from build123d import *

# Parameters (mm, degrees)
EXTRUDE_1_DEPTH     = 77
SKETCH_2_R          = 1.75
CUT_EXTRUDE_1_DEPTH = 20
SKETCH_3_W          = 6
SKETCH_3_H          = 3
CUT_EXTRUDE_2_DEPTH = 84.228292678
SKETCH_4_R          = 13.25
CUT_EXTRUDE_3_DEPTH = 84.228292678
SKETCH_7_R          = 1.75
CUT_EXTRUDE_4_DEPTH = 84.228292822


with BuildPart() as part:
    # Эскиз1 → Бобышка-Вытянуть1 (new body)
    with BuildSketch(Plane(origin=(0, 0, 0), x_dir=(-1, 0, 0), z_dir=(0, 1, 0))):
        with BuildLine():
            Line((27.5, 9.103890562), (20.77355029, -2.54666209))
            ThreePointArc((20.77355029, -2.54666209), (0, 0), (-20.77355029, -2.54666209))
            Line((-20.77355029, -2.54666209), (-27.5, 9.103890562))
            ThreePointArc((-27.5, 9.103890562), (0, 13), (27.5, 9.103890562))
        make_face()
    extrude(amount=EXTRUDE_1_DEPTH)

    # Эскиз2 → Вырез-Вытянуть1 (cut)
    with BuildSketch(Plane.XZ):
        with Locations(Location((0, 6.5, 0), (0, 0, 270))):
            Circle(SKETCH_2_R)
        with Locations(Location((16.059644847, 5.07877185, 0), (0, 0, 270))):
            Circle(SKETCH_2_R)
        with Locations(Location((-16.059644847, 5.07877185, 0), (0, 0, 270))):
            Circle(SKETCH_2_R)
    extrude(amount=-CUT_EXTRUDE_1_DEPTH, mode=Mode.SUBTRACT)

    # Эскиз3 → Вырез-Вытянуть2 (cut, through all)
    with BuildSketch(Plane.XY.offset(13)):
        with Locations((-16.059644847, 11.5)):
            Rectangle(SKETCH_3_W, SKETCH_3_H)
        with Locations((0, 11.5)):
            Rectangle(SKETCH_3_W, SKETCH_3_H)
        with Locations((16.059644847, 11.5)):
            Rectangle(SKETCH_3_W, SKETCH_3_H)
    extrude(amount=-CUT_EXTRUDE_2_DEPTH, mode=Mode.SUBTRACT)

    # Эскиз4 → Вырез-Вытянуть3 (cut, through all)
    with BuildSketch(Plane.XY.offset(13)):
        with Locations((0, 44.5)):
            Circle(SKETCH_4_R)
    extrude(amount=-CUT_EXTRUDE_3_DEPTH, mode=Mode.SUBTRACT)

    # Эскиз7 → Вырез-Вытянуть4 (cut, through all)
    with BuildSketch(Plane.XY.offset(13)):
        with Locations((-17.5, 62)):
            Circle(SKETCH_7_R)
        with Locations((17.5, 62)):
            Circle(SKETCH_7_R)
        with Locations((17.5, 27)):
            Circle(SKETCH_7_R)
        with Locations((-17.5, 27)):
            Circle(SKETCH_7_R)
    extrude(amount=-CUT_EXTRUDE_4_DEPTH, mode=Mode.SUBTRACT)


solid = part.part
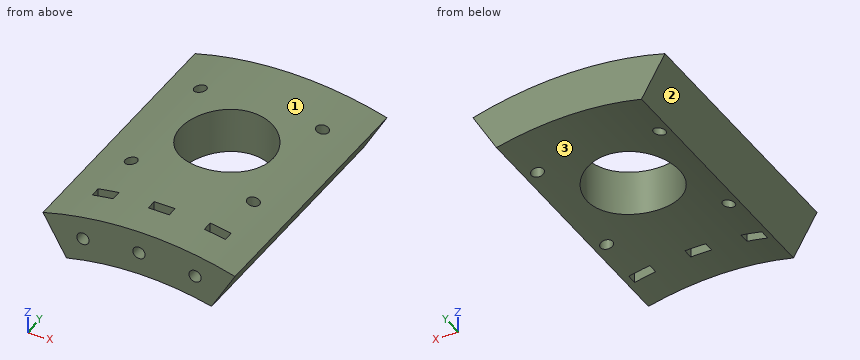
Part model, mm, in its own coordinate system. Face numbers are marked on the shaded views. Coordinates: 2 decimals unless noted, no trailing zeros. Order: outer loops, then holes, each group sorted by start corner. A loop starts at its lowest first (then second) coordinate and runs counter-clockwise, first axis right, second up.
(1) Pull direction X, two halves, no side cores. Call the marked faces 1, 2 and 3: pulls with the +X half, pulls with the -X half, needs draft (parallel to the pull), parting line crosses it, or undercut.
Check sheet entries:
face 1: parting line crosses it
face 2: pulls with the -X half
face 3: undercut
(2) Slice it at D-D, the plane z = 1.5. State how many separate pieces and enclosed holes the cut face has, and give its area (3 significant figures).
Check sheet entries:
separate pieces: 1
enclosed holes: 8
area: 2,910 mm2
(3) Slice it at A-A, the plane x = 0. Write the cut outline in (y, z).
Check sheet entries:
outline: (0, 0) - (10, 0) - (10, 4.75) - (0, 4.75) - close; (0, 8.25) - (10, 8.25) - (10, 13) - (0, 13) - close; (13, 0) - (31.25, 0) - (31.25, 13) - (13, 13) - (13, 8.25) - (20, 8.25) - (20, 4.75) - (13, 4.75) - close; (57.75, 0) - (77, 0) - (77, 13) - (57.75, 13) - close
(4) Probe L1, parallel to Y at x = -13.5, z = 2.75; L2, parallel to X at y = 13.5, z = 5.25; L3, parallel to Y at x = 18, z = 2.25. List the from-to ranges inside material, lowest first.
Check sheet entries:
L1: y = 0 to 10, 13 to 77
L2: x = -25.27 to -17.8, -14.32 to -1.22, 1.22 to 14.32, 17.8 to 25.27
L3: y = 0 to 10, 13 to 25.32, 28.68 to 60.32, 63.68 to 77
(5) Slice it at B-B, the plane y = 62. Write the cut outline in (x, z), and give its area (3 significant figures).
Check sheet entries:
outline: (-27.5, 9.1) - (-20.77, -2.55) arc R86 cw to (-19.25, -2.18) - (-19.25, 11.11) arc R99 ccw to start; (-15.75, -1.45) arc R86 cw to (15.75, -1.45) - (15.75, 11.74) arc R99 ccw to (-15.75, 11.74) - close; (19.25, -2.18) arc R86 cw to (20.77, -2.55) - (27.5, 9.1) arc R99 ccw to (19.25, 11.11) - close
area: 542 mm2
(6) Slice it at C-C, the plane x = -17. Write the cut outline in (y, z), and give its area (3 significant figures).
Check sheet entries:
outline: (0, -1.7) - (10, -1.7) - (10, 3.6) - (0, 3.6) - close; (0, 6.55) - (10, 6.55) - (10, 11.53) - (0, 11.53) - close; (13, -1.7) - (25.32, -1.7) - (25.32, 11.53) - (13, 11.53) - (13, 6.55) - (20, 6.55) - (20, 3.6) - (13, 3.6) - close; (28.68, -1.7) - (60.32, -1.7) - (60.32, 11.53) - (28.68, 11.53) - close; (63.68, -1.7) - (77, -1.7) - (77, 11.53) - (63.68, 11.53) - close
area: 840 mm2
(7) Pin check, flat tips, straight feed: pin 1 Ø1.5 at (y, z) = (11, 5) entering from -X; pin 2 Ø3 at (x, y) = (17.5, 62) entering from +Z; pin 3 Ø5 at (y, z) = (39, 0) entering from -X; pin 4 Ø1 at (x, z) = (-1, 6) entering from -Y. Stop position of each tip, or through.
Check sheet entries:
pin 1: stops at x = -25.56
pin 2: passes through
pin 3: stops at x = -23.69
pin 4: stops at y = 20
